Solid Edge part; units mm, degrees
sketch "Sketch1" plane through (0, 0, 0) normal (0, 0, 1) x (1, 0, 0)
  line L0 (10, -10) -> (10, 10)
  line L1 (10, 10) -> (-10, 10)
  line L2 (-10, 10) -> (-10, -10)
  line L3 (-10, -10) -> (10, -10)
extrude "Protrusion1" add sketch "Sketch1" along normal blind 73.108
sketch "Sketch2" plane through (0, 0, 0) normal (1, 0, 0) x (0, 1, 0)
  line L0 (0, 14.1421) -> (10, 0)
extrude "Cutout1" cut sketch "Sketch2" along normal up to next and the other way up to next material side at (0, 5.0408, 7.0999)
pattern_circular "Pattern1" count 4 over 360 about axis through (0, 0, 0) along (0, 0, 1) of "Cutout1"
The listing builds one solid part. Answer for the finished solid, in the listing's coordinates (mm). Coordinates: 2 decimals unless noted, no trailing zeros. Write each loop counter-clockwise with the first axis right and the second up, starting at its lowest first coordinate (ties: lowest second). Pieces come first, ordered by that corner, then holes. Notation, with made-up numbers: M 65.25,34 L 72.25,34 A27 ccw 72.25,67 Z; hole C 9.5,65 d4. An arc over 180 degrees is marked long. Use a Markdown table: item, result. Add a question column.
1. Straight lines are drawn through the part: line 1 along X through (y, z) = (-1.5, 8.75); line 2 along Z through (x, y) = (6.25, -3.5); line 3 along X through (y, z) = (-1, 4.25). For each, find the intervals that lie inside material, in ascending order. Write a range as [from, to].
2. Section B-B (x = 5.5) is taken. Give the vertices of the cut face in (y, z), plus the area to 3 significant figures.
3. Given P1, Ø8, axis at y = -6.5, z = 11, coming from the +X side; P2, Ø8, axis at x = 5.5, z = 7, coming from the -Y side; P3, Ø6, axis at x = -3.5, y = 5.5, coming from the +Z side, each flat-ended and moving along its own axis, determine where each tip first touches the part or whether it passes through.
4. Section A-A (z = 1.25) is taken. Give the vertices of the cut face in (x, y), plus the area to 3 significant figures.
Data:
| question | item | result |
|---|---|---|
| 1 | line 1 | x = [-3.81, 3.81] |
| 1 | line 2 | z = [0, 5.3] |
| 1 | line 3 | x = [-6.99, 6.99] |
| 2 | outline | M -10,0 L 10,0 L 5.5,6.36 L -5.5,6.36 Z |
| 2 | area | 98.6 mm2 |
| 3 | P1 | stops at x = 4.77 |
| 3 | P2 | stops at y = -7.88 |
| 3 | P3 | stops at z = 10.42 |
| 4 | outline | M -9.12,-9.12 L 9.12,-9.12 L 9.12,9.12 L -9.12,9.12 Z |
| 4 | area | 332 mm2 |
